```python
from build123d import *

# Parameters (mm, degrees)
SKETCH1_R               = 30
BOSS_EXTRUDE1_DEPTH     = 10
SKETCH2_R               = 2.5
CUT_EXTRUDE1_DEPTH      = 44.588989435
SKETCH5_R               = 14
BOSS_EXTRUDE4_DEPTH     = 6
SKETCH8_R               = 15
BOSS_EXTRUDE6_DEPTH     = 1
SKETCH13_R              = 15
BOSS_EXTRUDE7_DEPTH     = 10
CUT_EXTRUDE4_REACH      = 52.289
SKETCH14_R              = 7.5
CUT_EXTRUDE3_REACH      = 60.017
CUT_EXTRUDE3_END_RADIUS = 7.5
SKETCH12_R              = 3


with BuildPart() as part:
    # Sketch1 → Boss-Extrude1 (new body)
    with BuildSketch(Plane(origin=(0, 0, 0), x_dir=(0, 0, -1), z_dir=(1, 0, 0))):
        Circle(SKETCH1_R)
    extrude(amount=BOSS_EXTRUDE1_DEPTH)

    # Sketch2 → Cut-Extrude1 (cut, through all)
    with BuildSketch(Plane(origin=(10, 0, 0), x_dir=(0, 0, -1), z_dir=(1, 0, 0))):
        with Locations((0, 23.75)):
            Circle(SKETCH2_R)
        with Locations((20.56810334, 11.875)):
            Circle(SKETCH2_R)
        with Locations((20.56810334, -11.875)):
            Circle(SKETCH2_R)
        with Locations((0, -23.75)):
            Circle(SKETCH2_R)
        with Locations((-20.56810334, -11.875)):
            Circle(SKETCH2_R)
        with Locations((-20.56810334, 11.875)):
            Circle(SKETCH2_R)
    extrude(amount=-CUT_EXTRUDE1_DEPTH, mode=Mode.SUBTRACT)

    # Sketch5 → Boss-Extrude4 (add)
    with BuildSketch(Plane.ZY):
        with Locations(Location((0, 0, 0), (0, 0, 180))):
            Circle(SKETCH5_R)
    extrude(amount=BOSS_EXTRUDE4_DEPTH)

    # Sketch8 → Boss-Extrude6 (add)
    with BuildSketch(Plane(origin=(10, 0, 0), x_dir=(0, 0, -1), z_dir=(1, 0, 0))):
        Circle(SKETCH8_R)
    extrude(amount=BOSS_EXTRUDE6_DEPTH)

    # Sketch13 → Boss-Extrude7 (add)
    with BuildSketch(Plane(origin=(11, 0, 0), x_dir=(0, 0, -1), z_dir=(1, 0, 0))):
        Circle(SKETCH13_R)
    extrude(amount=BOSS_EXTRUDE7_DEPTH)

    # Sketch14 → Cut-Extrude4 (cut, up to next)
    with BuildSketch(Plane(origin=(21, 0, 0), x_dir=(0, 0, -1), z_dir=(1, 0, 0)), mode=Mode.PRIVATE) as cut_extrude4_sk1:
        Circle(SKETCH14_R)
    cut_extrude4_tool1 = extrude(cut_extrude4_sk1.sketch, amount=-CUT_EXTRUDE4_REACH, mode=Mode.PRIVATE) & part.part
    add(cut_extrude4_tool1.solids().sort_by_distance((21, 0, 0))[0], mode=Mode.SUBTRACT)

    # Cut-Extrude3: up to this cylinder (the profile starts outside it)
    cut_extrude3_end = Plane(origin=(16, 0, 0), z_dir=(1, 0, 0)) * Cylinder(CUT_EXTRUDE3_END_RADIUS, 136.034, mode=Mode.PRIVATE)
    # Sketch12 → Cut-Extrude3 (cut, up to the surface)
    with BuildSketch(Plane(origin=(0, -15, 0), x_dir=(-1, 0, 0), z_dir=(0, -1, 0)), mode=Mode.PRIVATE) as cut_extrude3_sk1:
        with Locations(Location((-16, 0, 0), (0, 0, 90))):
            Circle(SKETCH12_R)
    cut_extrude3_tool1 = extrude(cut_extrude3_sk1.sketch, amount=-CUT_EXTRUDE3_REACH, mode=Mode.PRIVATE) - cut_extrude3_end
    add(cut_extrude3_tool1.solids().sort_by_distance((16, -15, 0))[0], mode=Mode.SUBTRACT)


solid = part.part
```
Can you work these out from the model? Positions are in its coordinate system, mm. A direction names the side the tool comes from. Give positions to 0.01 mm unless a question says otherwise; leave off trailing zeros. Write each loop counter-clockwise with the first axis right and the second up, starting at its lowest first coordinate (ties: lowest second). Pieces come first, ordered by that corner, then holes. Notation, with made-up numbers: (67, 74) -> (118, 74) arc R22 cw to (118, 100) -> close; hole circle Ø9 at (50, 0). An arc over 180 degrees is marked (long way). One line per item, written item: value.
Q1. Imagine slicing it at C-C on z = -21. Please give me the cut outline in (x, y), and give its area (3 significant figures).
Results found:
outline: (0, -21.42) -> (10, -21.42) -> (10, -14.34) -> (0, -14.34) -> close; (0, -9.41) -> (10, -9.41) -> (10, 9.41) -> (0, 9.41) -> close; (0, 14.34) -> (10, 14.34) -> (10, 21.42) -> (0, 21.42) -> close
area: 330 mm^2
Q2. Imagine slicing it at A-A on y = 0. Please give me the cut outline in (x, z), and give its area (3 significant figures).
Results found:
outline: (-6, -14) -> (0, -14) -> (0, -30) -> (10, -30) -> (10, -15) -> (21, -15) -> (21, -7.5) -> (-6, -7.5) -> close; (-6, 7.5) -> (21, 7.5) -> (21, 15) -> (10, 15) -> (10, 30) -> (0, 30) -> (0, 14) -> (-6, 14) -> close
area: 693 mm^2
Q3. Imagine slicing it at D-D on x = 6. Please give me the cut outline in (y, z) (3 decimals), and give its area (3 significant figures).
Results found:
outline: circle Ø60 at (0, 0); hole circle Ø5 at (-23.75, 0); hole circle Ø5 at (-11.875, -20.568); hole circle Ø5 at (-11.875, 20.568); hole circle Ø15 at (0, 0); hole circle Ø5 at (11.875, -20.568); hole circle Ø5 at (11.875, 20.568); hole circle Ø5 at (23.75, 0)
area: 2,530 mm^2
Q4. Please list where these lines run through material, in increasing order: line 1 (Y direction, x = 5.75, z = 0); line 2 (Y direction, x = 1, z = -19.5); line 3 (X direction, y = -20, z = 18.5). Write a range as [from, to].
Results found:
line 1: y = [-30, -26.25], [-21.25, -7.5], [7.5, 21.25], [26.25, 30]
line 2: y = [-22.8, -14.14], [-9.61, 9.61], [14.14, 22.8]
line 3: x = [0, 10]
Q5. For P1, Ø6.5, axis at y = -23.75, z = 0, coming from the -X side; P2, Ø12, axis at y = 0, z = 0, coming from the +X side; P3, Ø4, axis at y = 16, z = -9, coming from the +X side; P4, Ø1.5, axis at x = 2, z = 9, coming from the +Y side, each with a flat end and sliding along its axis, tell me the tip position at first contact or that it passes through.
Results found:
P1: stops at x = 0
P2: passes through
P3: stops at x = 10
P4: stops at y = 28.84
Q6. Which directions (+Z, -Z, +X, -X, +Y, -Y) give clear straight access to the entire face, cutting with the end or side of a thin tool? Please do faces 1 (the face through (5.07, 9.657, -21.722)), 2 (the face through (-2.958, 5.362, -12.932)), 3 (the face through (15.423, 0.66, 14.985)).
Results found:
face 1: +X, -X
face 2: -X
face 3: +X
Q7. We'd pull the mould along X, two halves only. Please class faces 4 (the face through (14.85, -10.99, -2.77)), 5 (the face through (5.07, 26.23, 0.33)), 6 (the face through (21, 7, 4)): +X half, -X half, draft (parallel to the pull), parting line (faces both ways), or undercut.
Results found:
face 4: undercut
face 5: draft
face 6: +X half
Q8. Imagine slicing it at B-B on z = 0. Please give me the cut outline in (x, y).
Results found:
outline: (-6, -14) -> (0, -14) -> (0, -21.25) -> (10, -21.25) -> (10, -15) -> (13, -15) -> (13, -7.5) -> (-6, -7.5) -> close; (-6, 7.5) -> (21, 7.5) -> (21, 15) -> (10, 15) -> (10, 21.25) -> (0, 21.25) -> (0, 14) -> (-6, 14) -> close; (0, -30) -> (10, -30) -> (10, -26.25) -> (0, -26.25) -> close; (0, 26.25) -> (10, 26.25) -> (10, 30) -> (0, 30) -> close; (19, -15) -> (21, -15) -> (21, -7.5) -> (19, -7.5) -> close
